```python
from build123d import *

# Parameters (mm, degrees)
CUT_EXTRUDE1_DEPTH      = 21
CUT_EXTRUDE2_DEPTH      = 19.547236991
CUT_EXTRUDE2_DEPTH_BACK = 19.547236991
SKETCH6_R               = 1


with BuildPart() as part:
    # Sketch4 → Revolve1 (revolve)
    with BuildSketch(Plane.XY, mode=Mode.PRIVATE) as revolve1_sk:
        Polygon((0, 0), (10, 0), (10, 1.289403445), (9.090035529, 2.199367917), (9.090035529, 7.199367917), (10, 8.109332388), (10, 9), (6.735647112, 9), (6, 12), (0, 12), (0, 9), align=None)
    revolve(revolve1_sk.sketch.rotate(Axis((0, 9, 0), (0, -1, 0)), 90), axis=Axis((0, 9, 0), (0, -1, 0)))

    # Sketch5 → Cut-Extrude1 (cut)
    with BuildSketch(Plane(origin=(0, 12, 0), x_dir=(1, 0, 0), z_dir=(0, 1, 0))):
        with BuildLine():
            Line((1.9375, 3.35584844), (-1.9375, 3.35584844))
            ThreePointArc((-1.9375, 3.35584844), (-3.875, 0), (-1.9375, -3.35584844))
            Line((-1.9375, -3.35584844), (1.9375, -3.35584844))
            ThreePointArc((1.9375, -3.35584844), (3.875, 0), (1.9375, 3.35584844))
        make_face()
    extrude(amount=-CUT_EXTRUDE1_DEPTH, mode=Mode.SUBTRACT)

    # Sketch6 → Cut-Extrude2 (cut, two sides: drawn at the far end of the back side and taken through both)
    with BuildSketch(Plane.XY.offset(-CUT_EXTRUDE2_DEPTH_BACK)):
        with Locations((0, 5)):
            Circle(SKETCH6_R)
    extrude(amount=CUT_EXTRUDE2_DEPTH + CUT_EXTRUDE2_DEPTH_BACK, mode=Mode.SUBTRACT)


solid = part.part
```
Could you check a few things on this model? Use its own coordinates, in mm. A direction names the side the tool comes from. Round coordinates to 2 decimals unless told otherwise and drop trailing zeros. Loops run counter-clockwise (first coordinate to the right, second up) from the corner with the lowest first, then second, coordinate; pieces in that order, holes last. Notation, with made-up numbers: (44, 49.25) - (51, 49.25) arc R18 ccw to (51, 61.25) - close; hole circle Ø1 at (61, 8). An arc over 180 degrees is marked (long way). Answer in a Markdown table with one row per item. Add a question column.
(1) I'm going to push flat-ended pins straight in: pin 1 (6 mm diameter, centred on y = 2, z = -5, fed in from +X); pin 2 (2.5 mm diameter, centred on x = 0, y = 5, fed in from -Z); pin 3 (3 mm diameter, centred on x = 1.5, y = 2, fed in from -Z). Where does each tip first touch, or does it pass through?
(2) I need wall thicknesses on line 1 along Y through (x, z) = (0, 5.5); line 2 along X through (y, z) = (5.5, 7); line 3 along X through (y, z) = (5, -1.25). Which ranges of each line are inside material? Lowest first, please.
(3) If we section it at A-A (x = 0): Please give me the cut outline in (y, z), plus the area to 3 significant figures.
(4) If we section it at C-C (z = 0): Please give me the cut outline in (x, y) (3 decimals).
(5) If we mould it in two halves opening along X, with no side actions, what happens to faces 6 (the face through (0, 0, -4)), 7 (the face through (-3.875, 6.084, -0.057)), 8 (the face through (0, 1, -10))? For each: pulls with the +X half, pulls with the -X half, needs draft (parallel to the pull), parting line crosses it, or undercut.
(6) For faces 1 (the face through (0, 12, 4)), 2 (the face through (0, 6, 6)), 3 (the face through (3.875, 6.084, 0.057)), 4 (the face through (2, 9, 7)), 5 (the face through (-2.73, 4.73, 8.67)), which set-ups out of +Z, -Z, +X, -X, +Y, -Y let a thin tool reach every point of the face, with its end or its side?
Model answer:
| question | item | result |
|---|---|---|
| 1 | pin 1 | stops at x = 9.78 |
| 1 | pin 2 | stops at z = -9.09 |
| 1 | pin 3 | stops at z = -10 |
| 2 | line 1 | y = 0 to 4, 6 to 12 |
| 2 | line 2 | x = -5.8 to -0.87, 0.87 to 5.8 |
| 2 | line 3 | x = -9 to -3.67, 3.67 to 9 |
| 3 | outline | (0, -10) - (1.29, -10) - (2.2, -9.09) - (4, -9.09) - (4, -3.36) - (0, -3.36) - close; (0, 3.36) - (4, 3.36) - (4, 9.09) - (2.2, 9.09) - (1.29, 10) - (0, 10) - close; (6, -9.09) - (7.2, -9.09) - (8.11, -10) - (9, -10) - (9, -6.74) - (12, -6) - (12, -3.36) - (6, -3.36) - close; (6, 3.36) - (12, 3.36) - (12, 6) - (9, 6.74) - (9, 10) - (8.11, 10) - (7.2, 9.09) - (6, 9.09) - close |
| 3 | area | 104 mm² |
| 4 | outline | (-10, 0) - (-3.875, 0) - (-3.875, 12) - (-6, 12) - (-6.736, 9) - (-10, 9) - (-10, 8.109) - (-9.09, 7.199) - (-9.09, 2.199) - (-10, 1.289) - close; (3.875, 0) - (10, 0) - (10, 1.289) - (9.09, 2.199) - (9.09, 7.199) - (10, 8.109) - (10, 9) - (6.736, 9) - (6, 12) - (3.875, 12) - close |
| 5 | face 6 | needs draft |
| 5 | face 7 | undercut |
| 5 | face 8 | parting line crosses it |
| 6 | face 1 | +Z, -Z, +X, -X, +Y |
| 6 | face 2 | +Z, -Z |
| 6 | face 3 | +Y, -Y |
| 6 | face 4 | +Y |
| 6 | face 5 | none |
